```python
from build123d import *

# Parameters (mm, degrees)
SZKIC1_R                    = 6
DODANIE_WYCI_GNI_CIE3_DEPTH = 3
SZKIC2_R                    = 6
DODANIE_WYCI_GNI_CIE5_DEPTH = 3
SZKIC3_R                    = 12
DODANIE_WYCI_GNI_CIE7_DEPTH = 12
SZKIC4_R                    = 3
WYTNIJ_WYCI_GNI_CIE1_DEPTH  = 6
SZKIC5_R                    = 6
WYTNIJ_WYCI_GNI_CIE2_DEPTH  = 6


with BuildPart() as part:
    # Szkic1 → Dodanie-wyciągnięcie3 (new body)
    with BuildSketch(Plane(origin=(0, 0, 0), x_dir=(1, 0, 0), z_dir=(0, 1, 0))):
        with BuildLine():
            ThreePointArc((18.846153454, 38.65), (16.147655157, 40.973517523), (14.941453584, 44.323995772))
            ThreePointArc((14.941453584, 44.323995772), (0, 58), (-14.941453584, 44.323995772))
            ThreePointArc((-14.941453584, 44.323995772), (-16.147655157, 40.973517523), (-18.846153454, 38.65))
            ThreePointArc((-18.846153454, 38.65), (-37.579169087, 20.89990552), (-42.776535296, -4.378130663))
            ThreePointArc((-42.776535296, -4.378130663), (-43.223069571, -6.802925196), (-44.904285151, -8.606403934))
            ThreePointArc((-44.904285151, -8.606403934), (-50.503687636, -28.503607088), (-30.914979544, -35.101676259))
            ThreePointArc((-30.914979544, -35.101676259), (-27.410279478, -34.471038339), (-24.048805129, -35.646247655))
            ThreePointArc((-24.048805129, -35.646247655), (0, -43), (24.048805129, -35.646247655))
            ThreePointArc((24.048805129, -35.646247655), (27.410279478, -34.471038339), (30.914979544, -35.101676259))
            ThreePointArc((30.914979544, -35.101676259), (50.229473419, -29), (45.856433127, -9.222319513))
            ThreePointArc((45.856433127, -9.222319513), (43.557934635, -6.502479184), (42.894958583, -3.003752345))
            ThreePointArc((42.894958583, -3.003752345), (37.239092363, 21.5), (18.846153454, 38.65))
        make_face()
        with Locations(Location((0, 43, 0), (0, 0, 270))):
            Circle(SZKIC1_R, mode=Mode.SUBTRACT)
        with Locations(Location((37.239092363, -21.5, 0), (0, 0, 270))):
            Circle(SZKIC1_R, mode=Mode.SUBTRACT)
        with Locations(Location((-37.239092363, -21.5, 0), (0, 0, 270))):
            Circle(SZKIC1_R, mode=Mode.SUBTRACT)
    extrude(amount=DODANIE_WYCI_GNI_CIE3_DEPTH)

    # Szkic2 → Dodanie-wyciągnięcie5 (add)
    with BuildSketch(Plane(origin=(0, 3, 0), x_dir=(1, 0, 0), z_dir=(0, 1, 0))):
        with BuildLine():
            ThreePointArc((32.179802107, -32.381341007), (27.173087728, -31.480429693), (22.370981516, -33.159300144))
            ThreePointArc((22.370981516, -33.159300144), (0, -40), (-22.370981516, -33.159300144))
            ThreePointArc((-22.370981516, -33.159300144), (-27.173087728, -31.480429693), (-32.179802107, -32.381341007))
            ThreePointArc((-32.179802107, -32.381341007), (-47.850768581, -27.10288567), (-43.371246594, -11.185123147))
            ThreePointArc((-43.371246594, -11.185123147), (-40.543248024, -8.151463841), (-39.792125856, -4.072679686))
            ThreePointArc((-39.792125856, -4.072679686), (-34.957366592, 19.441772577), (-17.531305538, 35.953488372))
            ThreePointArc((-17.531305538, 35.953488372), (-13.676307972, 39.272799119), (-11.953162867, 44.059196617))
            ThreePointArc((-11.953162867, 44.059196617), (0, 55), (11.953162867, 44.059196617))
            ThreePointArc((11.953162867, 44.059196617), (13.676307972, 39.272799119), (17.531305538, 35.953488372))
            ThreePointArc((17.531305538, 35.953488372), (34.641016151, 20), (39.902287054, -2.794188228))
            ThreePointArc((39.902287054, -2.794188228), (40.8493957, -7.792369426), (44.132964974, -11.67785561))
            ThreePointArc((44.132964974, -11.67785561), (47.631397208, -27.5), (32.179802107, -32.381341007))
        make_face()
        with Locations(Location((37.239092363, -21.5, 0), (0, 0, 270))):
            Circle(SZKIC2_R, mode=Mode.SUBTRACT)
        with Locations(Location((0, 43, 0), (0, 0, 270))):
            Circle(SZKIC2_R, mode=Mode.SUBTRACT)
        with Locations(Location((-37.239092363, -21.5, 0), (0, 0, 270))):
            Circle(SZKIC2_R, mode=Mode.SUBTRACT)
    extrude(amount=DODANIE_WYCI_GNI_CIE5_DEPTH)

    # Szkic3 → Dodanie-wyciągnięcie7 (add)
    with BuildSketch(Plane(origin=(0, 6, 0), x_dir=(1, 0, 0), z_dir=(0, 1, 0))):
        with Locations(Location((0, 43, 0), (0, 0, 5.063881306))):
            Circle(SZKIC3_R)
        with Locations(Location((37.239092363, -21.5, 0), (0, 0, 54.936118694))):
            Circle(SZKIC3_R)
        with Locations(Location((-37.239092363, -21.5, 0), (0, 0, 120.73131892))):
            Circle(SZKIC3_R)
    extrude(amount=DODANIE_WYCI_GNI_CIE7_DEPTH)

    # Szkic4 → Wytnij-wyciągnięcie1 (cut)
    with BuildSketch(Plane(origin=(0, 18, 0), x_dir=(1, 0, 0), z_dir=(0, 1, 0))):
        with Locations(Location((0, 43, 0), (0, 0, 270))):
            Circle(SZKIC4_R)
        with Locations(Location((37.239092363, -21.5, 0), (0, 0, 270))):
            Circle(SZKIC4_R)
        with Locations(Location((-37.239092363, -21.5, 0), (0, 0, 270))):
            Circle(SZKIC4_R)
    extrude(amount=-WYTNIJ_WYCI_GNI_CIE1_DEPTH, mode=Mode.SUBTRACT)

    # Szkic5 → Wytnij-wyciągnięcie2 (cut)
    with BuildSketch(Plane.XZ.offset(-6)):
        with Locations(Location((37.239092363, 21.5, 0), (0, 0, 270))):
            Circle(SZKIC5_R)
        with Locations(Location((0, -43, 0), (0, 0, 270))):
            Circle(SZKIC5_R)
        with Locations(Location((-37.239092363, 21.5, 0), (0, 0, 270))):
            Circle(SZKIC5_R)
    extrude(amount=-WYTNIJ_WYCI_GNI_CIE2_DEPTH, mode=Mode.SUBTRACT)


solid = part.part
```
Input: part model. Units: mm. Frame: model coordinates. A direction names the side the tool comes from. Round coordinates to 2 decimals unless told otherwise and drop trailing zeros. Loops run counter-clockwise (first coordinate to the right, second up) from the corner with the lowest first, then second, coordinate; pieces in that order, holes last. Notation, with made-up numbers: (53.5, 39) -> (67.5, 39) arc R9 ccw to (67.5, 43) -> close; hole circle Ø3 at (-11.5, -18.5). An arc over 180 degrees is marked (long way). One line per item, written item: value.
(1) Pin query (flat end, axial travel): pin 1 (3.5 mm diameter, centred on x = -37.24, z = 21.5, fed in from -Y); pin 2 (8 mm diameter, centred on x = -10.5, y = 7.5, fed in from -Z); pin 3 (9.5 mm diameter, centred on x = 37.24, z = 21.5, fed in from +Y); pin 4 (3.5 mm diameter, centred on x = -2, z = -43.5, fed in from -Y). Return the tip coordinate at first contact, or that it passes through.
Geometry check:
pin 1: through
pin 2: z = -53.09
pin 3: y = 18
pin 4: y = 12
(2) Section B-B (z = 21.5). Return the cut outline in (x, y), plus the area to 3 significant figures.
Geometry check:
outline: (-52.24, 0) -> (-43.24, 0) -> (-43.24, 12) -> (-40.24, 12) -> (-40.24, 18) -> (-49.24, 18) -> (-49.24, 3) -> (-52.24, 3) -> close; (-34.24, 12) -> (-31.24, 12) -> (-31.24, 0) -> (31.24, 0) -> (31.24, 12) -> (34.24, 12) -> (34.24, 18) -> (25.24, 18) -> (25.24, 6) -> (-25.24, 6) -> (-25.24, 18) -> (-34.24, 18) -> close; (40.24, 12) -> (43.24, 12) -> (43.24, 0) -> (52.24, 0) -> (52.24, 3) -> (49.24, 3) -> (49.24, 18) -> (40.24, 18) -> close
area: 825 mm2
(3) Mould query, pull axis Z, two halves, no side actions, for faces 1 (the face through (1, 6, -3)), 2 (the face through (13.636, 4.479, -39.332)), 3 (the face through (-50.65, 1.48, 28.22)), 4 (the face through (38.7, 12, 24.3)). Classes: pulls with the +Z half, pulls with the -Z half, needs draft (parallel to the pull), parting line crosses it, or undercut.
Geometry check:
face 1: needs draft
face 2: pulls with the -Z half
face 3: parting line crosses it
face 4: undercut
(4) Material intervals for line 1 (X direction, y = 15.5, z = 21.5); line 2 (X direction, y = 16.6, z = -43); line 3 (Y direction, x = 6, z = -19), sorted ascending. Write a range as [from, to].
Geometry check:
line 1: [-49.24, -40.24], [-34.24, -25.24], [25.24, 34.24], [40.24, 49.24]
line 2: [-12, -3], [3, 12]
line 3: [0, 6]
(5) Section D-D (y = 1.5). Return the cut outline in (x, z).
Geometry check:
outline: (-44.9, 8.61) arc R4.4 cw to (-42.78, 4.38) arc R43 ccw to (-18.85, -38.65) arc R7 cw to (-14.94, -44.32) arc R15 ccw to (14.94, -44.32) arc R7 cw to (18.85, -38.65) arc R43 ccw to (42.89, 3) arc R7 cw to (45.86, 9.22) arc R15 ccw to (30.91, 35.1) arc R7 cw to (24.05, 35.65) arc R43 ccw to (-24.05, 35.65) arc R7 cw to (-30.91, 35.1) arc R15 ccw to start; hole circle Ø12 at (-37.24, 21.5); hole circle Ø12 at (0, -43); hole circle Ø12 at (37.24, 21.5)
(6) Section A-A (x = 0). Return the cut outline in (y, z), plus the area to 3 significant figures.
Geometry check:
outline: (0, -58) -> (3, -58) -> (3, -55) -> (18, -55) -> (18, -46) -> (12, -46) -> (12, -49) -> (0, -49) -> close; (0, -37) -> (12, -37) -> (12, -40) -> (18, -40) -> (18, -31) -> (6, -31) -> (6, 40) -> (3, 40) -> (3, 43) -> (0, 43) -> close
area: 696 mm2
(7) Section C-C (y = 7.5). Return the cut outline in (x, z), plus the area to 3 significant figures.
Geometry check:
outline: circle Ø24 at (-37.24, 21.5); circle Ø24 at (0, -43); circle Ø24 at (37.24, 21.5); hole circle Ø12 at (-37.24, 21.5); hole circle Ø12 at (0, -43); hole circle Ø12 at (37.24, 21.5)
area: 1,020 mm2
(8) Set-up query: faces 5 (the face through (0, 4, 40)), 6 (the face through (3, 12, -44)), 7 (the face through (-13.72, 4.48, -39.21)), 8 (the face through (-40.57, 4.48, 8.2)), 9 (the face through (43.58, 1.48, 6.55)). Return all of +Z, -Z, +X, -X, +Y, -Y with unobstructed straight access to the full face (end or side cutting, diameter ignored); none if empty.
Geometry check:
face 5: +Z, +Y
face 6: -Y
face 7: -Z, -X, +Y
face 8: -X, +Y
face 9: +X, +Y, -Y
